```python
from build123d import *

# Parameters (mm, degrees)
SKETCH1_W               = 442
SKETCH1_H               = 90
BOSS_EXTRUDE1_DEPTH     = 5
SKETCH3_W               = 5
SKETCH3_H               = 25
CUT_EXTRUDE2_DEPTH      = 226.590336672
SKETCH5_W               = 5
SKETCH5_H               = 30
BOSS_EXTRUDE2_DEPTH     = 5
SKETCH6_W               = 5
SKETCH6_H               = 20
CUT_EXTRUDE4_DEPTH      = 4
SKETCH7_R               = 1
CUT_EXTRUDE5_DEPTH      = 231.490780727
SKETCH8_W               = 20.2
SKETCH8_H               = 10
CUT_EXTRUDE6_DEPTH      = 10
SKETCH9_W               = 20.2
SKETCH9_H               = 10
CUT_EXTRUDE7_DEPTH      = 300
MIRROR4_COPY_1_SKETCH_W = 20.2
MIRROR4_COPY_1_SKETCH_H = 10
MIRROR4_COPY_1_DEPTH    = 10


with BuildPart() as part:
    # Sketch1 → Boss-Extrude1 (new body)
    with BuildSketch(Plane.XY):
        Rectangle(SKETCH1_W, SKETCH1_H)
    extrude(amount=BOSS_EXTRUDE1_DEPTH)

    # Sketch3 → Cut-Extrude2 (cut, through all)
    with BuildSketch(Plane(origin=(0, 0, 0), x_dir=(-1, 0, 0), z_dir=(0, 0, -1))):
        with Locations((0, 17.5)):
            Rectangle(SKETCH3_W, SKETCH3_H)
        with Locations((0, -17.5)):
            Rectangle(SKETCH3_W, SKETCH3_H)
    extrude(amount=-CUT_EXTRUDE2_DEPTH, mode=Mode.SUBTRACT)

    # Sketch5 → Boss-Extrude2 (add)
    with BuildSketch(Plane(origin=(221, 0, 0), x_dir=(0, 0, -1), z_dir=(1, 0, 0))):
        with Locations((-2.5, 25)):
            Rectangle(SKETCH5_W, SKETCH5_H)
        with Locations((-2.5, -25)):
            Rectangle(SKETCH5_W, SKETCH5_H)
    boss_extrude2 = extrude(amount=BOSS_EXTRUDE2_DEPTH)

    # Sketch6 → Cut-Extrude4 (cut)
    with BuildSketch(Plane(origin=(226, 0, 0), x_dir=(0, 0, -1), z_dir=(1, 0, 0))):
        with Locations((-2.5, 25)):
            Rectangle(SKETCH6_W, SKETCH6_H)
        with Locations((-2.5, -25)):
            Rectangle(SKETCH6_W, SKETCH6_H)
    cut_extrude4 = extrude(amount=-CUT_EXTRUDE4_DEPTH, mode=Mode.SUBTRACT)

    # Mirror1: Boss-Extrude2, Cut-Extrude4 across plane
    add(boss_extrude2.mirror(Plane(origin=(0, 0, 0), x_dir=(0, 0, 1), z_dir=(1, 0, 0))))
    add(cut_extrude4.mirror(Plane(origin=(0, 0, 0), x_dir=(0, 0, 1), z_dir=(1, 0, 0))), mode=Mode.SUBTRACT)

    # Sketch7 → Cut-Extrude5 (cut, through all)
    with BuildSketch(Plane(origin=(0, 0, 0), x_dir=(-1, 0, 0), z_dir=(0, 0, -1))):
        with Locations((-221, 9)):
            Circle(SKETCH7_R)
        with Locations((-221, -9)):
            Circle(SKETCH7_R)
        with Locations((-221, -41)):
            Circle(SKETCH7_R)
        with Locations((221, -41)):
            Circle(SKETCH7_R)
        with Locations((221, -9)):
            Circle(SKETCH7_R)
        with Locations((221, 9)):
            Circle(SKETCH7_R)
        with Locations((-221, 41)):
            Circle(SKETCH7_R)
        with Locations((221, 41)):
            Circle(SKETCH7_R)
    extrude(amount=-CUT_EXTRUDE5_DEPTH, mode=Mode.SUBTRACT)

    # Sketch8 → Cut-Extrude6 (cut)
    with BuildSketch(Plane(origin=(102.718818309, -610.456150304, 5), x_dir=(1, 0, 0), z_dir=(0, 0, 1))):
        with Locations((93.281181691, 585.456150304)):
            Rectangle(SKETCH8_W, SKETCH8_H)
    cut_extrude6 = extrude(amount=-CUT_EXTRUDE6_DEPTH, mode=Mode.SUBTRACT)

    # Mirror2: Cut-Extrude6 across plane
    add(cut_extrude6.mirror(Plane(origin=(0, 0, 0), x_dir=(0, 0, 1), z_dir=(1, 0, 0))), mode=Mode.SUBTRACT)

    # Sketch9 → Cut-Extrude7 (cut)
    with BuildSketch(Plane(origin=(102.718818309, -610.456150304, 228.5), x_dir=(1, 0, 0), z_dir=(0, 0, 1))):
        with Locations((-130.118818309, 585.456150304)):
            Rectangle(SKETCH9_W, SKETCH9_H)
    cut_extrude7 = extrude(amount=-CUT_EXTRUDE7_DEPTH, mode=Mode.SUBTRACT)

    # Mirror3: Cut-Extrude7 across plane
    add(cut_extrude7.mirror(Plane(origin=(0, 0, 0), x_dir=(0, 0, 1), z_dir=(1, 0, 0))), mode=Mode.SUBTRACT)

    # Mirror4: Cut-Extrude6 across plane
    add(cut_extrude6.mirror(Plane.ZX.offset(3.5)), mode=Mode.SUBTRACT)

    # Mirror4 copy 1 sketch → Mirror4 copy 1 (cut)
    with BuildSketch(Plane(origin=(-102.718818309, 617.456150304, 5), x_dir=(-1, 0, 0), z_dir=(0, 0, 1))):
        with Locations((93.281181691, 585.456150304)):
            Rectangle(MIRROR4_COPY_1_SKETCH_W, MIRROR4_COPY_1_SKETCH_H)
    extrude(amount=-MIRROR4_COPY_1_DEPTH, mode=Mode.SUBTRACT)


solid = part.part
```
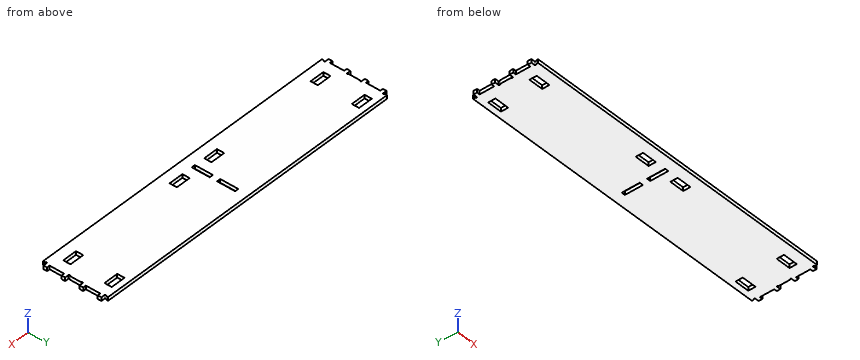
For this review, take the finished solid that the model builds, in its own axes (mm). Give positions to 0.01 mm unless a question says otherwise; leave off trailing zeros. Write each loop counter-clockwise with the first axis right and the second up, starting at its lowest first coordinate (ties: lowest second). Pieces come first, ordered by that corner, then holes. Notation, with made-up numbers: M 62,88 L 116,88 A29 ccw 116,111 Z; hole C 19,83 d3. An arc over 180 degrees is marked long. Answer as a JSON object with one key per item and string values. Group by question number.
Item 1: For probe 1 along X at (y, z) = (29, 4.4); probe 2 along X at (y, z) = (-25.5, 1.65); probe 3 along X at (y, z) = (16.5, 3.4), list the stretches that pass through material, from the lowest coordinate up. Write a range as [from, to].
Item 2: Consider section A-A on y = -24. Write out the cut boundary in (x, z), plus the area to 3 significant figures.
Item 3: For pin 1 Ø3 at (x, z) = (-224, 3) entering from -Y; pin 2 Ø1.5 at (x, z) = (-223.5, 2.5) entering from +Y; pin 3 Ø3 at (y, z) = (23, 4) entering from +X, all flat-tipped, find the tip position at first contact; note any pin that passes through.
Item 4: Consider section B-B on z = 2.6. Count the separate pieces of the cut face and the enclosed holes in it, plus the area to 3 significant figures.
Item 5: Consider section C-C on y = -1. Write out the cut boundary in (x, z).
Check result:
{
 "1": {"probe 1": "x = [-222, -206.1], [-185.9, -2.5], [2.5, 185.9], [206.1, 222]", "probe 2": "x = [-222, -206.1], [-185.9, -37.5], [-17.3, -2.5], [2.5, 17.3], [37.5, 185.9], [206.1, 222]", "probe 3": "x = [-222, -2.5], [2.5, 222]"},
 "2": {"outline": "M -222,0 L -206.1,0 L -206.1,5 L -222,5 Z; M -185.9,0 L -37.5,0 L -37.5,5 L -185.9,5 Z; M -17.3,0 L -2.5,0 L -2.5,5 L -17.3,5 Z; M 2.5,0 L 17.3,0 L 17.3,5 L 2.5,5 Z; M 37.5,0 L 185.9,0 L 185.9,5 L 37.5,5 Z; M 206.1,0 L 222,0 L 222,5 L 206.1,5 Z", "area": "1,790 mm^2"},
 "3": {"pin 1": "stops at y = -40", "pin 2": "stops at y = 40", "pin 3": "stops at x = 222"},
 "4": {"separate pieces": "1", "enclosed holes": "8", "area": "38,600 mm^2"},
 "5": {"outline": "M -221,0 L 221,0 L 221,5 L -221,5 Z"}
}
